The listing builds one solid part. Answer for the finished solid, in the listing's coordinates (mm). A direction names the side the tool comes from. Round coordinates to 2 decimals unless told otherwise and drop trailing zeros. Loops run counter-clockwise (first coordinate to the right, second up) from the corner with the lowest first, then second, coordinate; pieces in that order, holes last. Notation, with made-up numbers: (-18.5, 34.25) -> (39.5, 34.25) arc R30 cw to (39.5, 72.25) -> close; hole circle Ø1 at (29, -5). An arc over 180 degrees is marked (long way). Write each question's results on one line, items separated by ' | '. Start each with the question number.
(1) Flat-ended cylindrical pins translate along their axes: pin 1 (12 mm diameter, centred on x = -8.5, z = -67, fed in from -Y); pin 2 (1 mm diameter, centred on x = -8.5, y = 26.5, fed in from -Z); pin 3 (6 mm diameter, centred on y = 6, z = -101, fed in from +X); pin 4 (1 mm diameter, centred on y = 35.5, z = -7, fed in from -X). Find the tip coordinate at first contact, or state that the pin passes through.
(2) The part is cut by section B-B (z = 10). Determine the outline of the cut face in (x, y), plus the area to 3 significant figures.
(3) Straight lines are drawn through the part: probe 1 along Y at (x, z) = (-2.75, -100); probe 2 along Y at (x, z) = (-5, -95); probe 3 along Z at (x, y) = (-9.5, 39.5). For each, find the intervals that lie inside material, in ascending order.
(4) The part is cut by section C-C (y = 5). Determine the outline of the cut face in (x, z).
(5) The part is cut by section A-A (x = -11.25). Determine the outline of the cut face in (y, z).
(6) Determine the mould class of faces 1 (the face through (-8, 35, 0)), 2 (the face through (1, 68.4, -36)), 3 (the face through (-5, 53.4, -97)) for opening direction Y: released by +Y, released by -Y, zero draft, split by the parting line, or undercut.
(7) For faces 4 (the face through (-10, 34, 7)), 5 (the face through (-5, 15, -97)), 6 (the face through (-1.93, 10.19, 4.585)), 7 (the face through (-10, 61, -98)), determine the directions among +Z, -Z, +X, -X, +Y, -Y from which every point of the face is accessible in a straight line to the end or side of a thin tool.
(8) The part is cut by section D-D (y = 49). Determine the outline of the cut face in (x, z).
Autodesk Inventor part; units mm, degrees
ref_plane "YZ Plane" through (0, 0, 0) normal (1, 0, 0) x (0, 1, 0)
ref_plane "XZ Plane" through (0, 0, 0) normal (0, 1, 0) x (-1, 0, 0)
ref_plane "XY Plane" through (0, 0, 0) normal (0, 0, 1) x (1, 0, 0)
sketch "Sketch1" plane through (0, 0, 0) normal (0, 0, 1) x (1, 0, 0)
  circle A0 centre (-20, 34.2) radius 10 construction
  line L0 (0, 0) -> (0, 68.4)
  line L1 (0, 0) -> (-20, 0)
  line L2 (-20, 0) -> (-20, 68.4) construction
  line L3 (-20, 68.4) -> (0, 68.4)
  line L4 (-20, 68.4) -> (-20, 44.2)
  line L5 (-20, 0) -> (-20, 24.2)
  arc A1 (-20, 24.2) -> (-20, 44.2) centre (-20, 34.2) ccw
  point P0 (0, 34.2)
  dimension "d0" = 20
  dimension "d1" = 20
  dimension "d3" = 68.4
extrude "Extrusion1" add sketch "Sketch1" along normal blind 15
sketch "Sketch2" plane through (0, 0, 0) normal (1, 0, 0) x (0, 0, -1)
  line L0 (-15, 68.4) -> (-15, 44.2)
  line L1 (-15, 68.4) -> (105, 68.4)
  line L2 (105, 68.4) -> (105, 0)
  line L3 (105, 0) -> (-15, 0)
  line L4 (-15, 0) -> (-15, 68.4)
  point P0 (0, 0)
  dimension "d6" = 120
extrude "Extrusion2" add sketch "Sketch2" along normal blind 3
sketch "Sketch3" plane through (-20, 0, 0) normal (-1, 0, 0) x (0, 0, 1)
  circle A0 centre (10, 5) radius 2.5
  circle A1 centre (10, 63.4) radius 2.5
  line L0 (0, 0) -> (15, 0)
  line L1 (15, 24.2) -> (15, 0)
  line L2 (15, 68.4) -> (15, 44.2)
  line L3 (0, 68.4) -> (15, 68.4)
  dimension "d9" = 5
  dimension "d10" = 5
  dimension "d11" = 5
  dimension "d12" = 5
  dimension "d13" = 5
  dimension "d14" = 5
extrude "Extrusion3" cut sketch "Sketch3" against normal through all
sketch "Sketch4" plane through (3, 0, 0) normal (1, 0, 0) x (0, 0, -1)
  circle A0 centre (-10, 63.4) radius 2.5
  circle A1 centre (-10, 5) radius 2.5
  circle A2 centre (-10, 63.4) radius 2.5
  circle A3 centre (-10, 63.4) radius 7.5
  circle A4 centre (-10, 5) radius 7.5
  point P0 (0, 0)
  dimension "d18" = 15
  dimension "d19" = 15
extrude "Extrusion4" cut sketch "Sketch4" against normal blind 10 contours A0 | A1 | A3 | A4
sketch "Sketch6" plane through (0, 0, 0) normal (-1, 0, 0) x (0, 0, 1)
  line L0 (-105, 68.4) -> (4.4098, 68.4)
  line L1 (-105, 68.4) -> (-90, 68.4)
  line L2 (-90, 68.4) -> (-90, 53.4)
  line L3 (-90, 53.4) -> (-105, 53.4)
  line L4 (-105, 53.4) -> (-105, 68.4)
  line L5 (4.4098, 0) -> (-105, 0)
  line L6 (-105, 0) -> (-90, 0)
  line L7 (-90, 0) -> (-90, 15)
  line L8 (-90, 15) -> (-105, 15)
  line L9 (-105, 15) -> (-105, 0)
  point P0 (0, 0)
  dimension "d22" = 15
  dimension "d23" = 15
  dimension "d24" = 15
  dimension "d25" = 15
extrude "Extrusion5" add sketch "Sketch6" along normal blind 10
sketch "Sketch7" plane through (-10, 0, 0) normal (-1, 0, 0) x (0, 0, 1)
  circle A0 centre (-100, 63.4) radius 2.5
  circle A1 centre (-100, 5) radius 2.5
  line L0 (-90, 68.4) -> (-105, 68.4)
  line L1 (-105, 68.4) -> (-105, 53.4)
  line L2 (-105, 0) -> (-90, 0)
  point P0 (0, 0)
  dimension "d30" = 5
  dimension "d31" = 5
  dimension "d32" = 5
  dimension "d33" = 5
  dimension "d34" = 5
extrude "Extrusion6" cut sketch "Sketch7" against normal through all
sketch "Sketch8" plane through (3, 0, 0) normal (1, 0, 0) x (0, 0, -1)
  circle A0 centre (100, 5) radius 2.5
  circle A1 centre (100, 63.4) radius 2.5
  circle A2 centre (100, 5) radius 2.5
  circle A3 centre (100, 5) radius 7.5
  circle A4 centre (100, 63.4) radius 7.5
  point P0 (0, 0)
  dimension "d37" = 15
  dimension "d38" = 15
extrude "Extrusion7" cut sketch "Sketch8" against normal blind 3
properties part number "BP008" material "ABS Plastic"
Checked values:
1) pin 1: passes through | pin 2: stops at z = 0 | pin 3: stops at x = 0 | pin 4: stops at x = 0
2) outline: (-20, 0) -> (-7, 0) -> (-7, 2.5) -> (-20, 2.5) -> close; (-20, 7.5) -> (-7, 7.5) -> (-7, 12.5) -> (3, 12.5) -> (3, 55.9) -> (-7, 55.9) -> (-7, 60.9) -> (-20, 60.9) -> (-20, 44.2) arc R10 cw to (-20, 24.2) -> close; (-20, 65.9) -> (-7, 65.9) -> (-7, 68.4) -> (-20, 68.4) -> close | area: 1,040 mm2
3) probe 1: y = 0 to 2.5, 7.5 to 15, 53.4 to 60.9, 65.9 to 68.4 | probe 2: y = 0 to 15, 53.4 to 68.4 | probe 3: z = 0 to 15
4) outline: (-20, 0) -> (0, 0) -> (0, -90) -> (-10, -90) -> (-10, -97.5) -> (0, -97.5) -> (0, -92.5) -> (3, -92.5) -> (3, 2.5) -> (-7, 2.5) -> (-7, 7.5) -> (-20, 7.5) -> close; (-20, 12.5) -> (-7, 12.5) -> (-7, 15) -> (-20, 15) -> close; (-10, -105) -> (0, -105) -> (0, -102.5) -> (-10, -102.5) -> close
5) outline: (0, 0) -> (29.36, 0) -> (29.36, 15) -> (0, 15) -> close; (39.04, 0) -> (68.4, 0) -> (68.4, 15) -> (39.04, 15) -> close; hole circle Ø5 at (5, 10); hole circle Ø5 at (63.4, 10)
6) face 1: zero draft | face 2: released by +Y | face 3: undercut
7) face 4: +Z, -Z, -X | face 5: -Z, -X | face 6: +X | face 7: -Z, -X, +Y, -Y
8) outline: (-20, 0) -> (0, 0) -> (0, -105) -> (3, -105) -> (3, 15) -> (-20, 15) -> close
